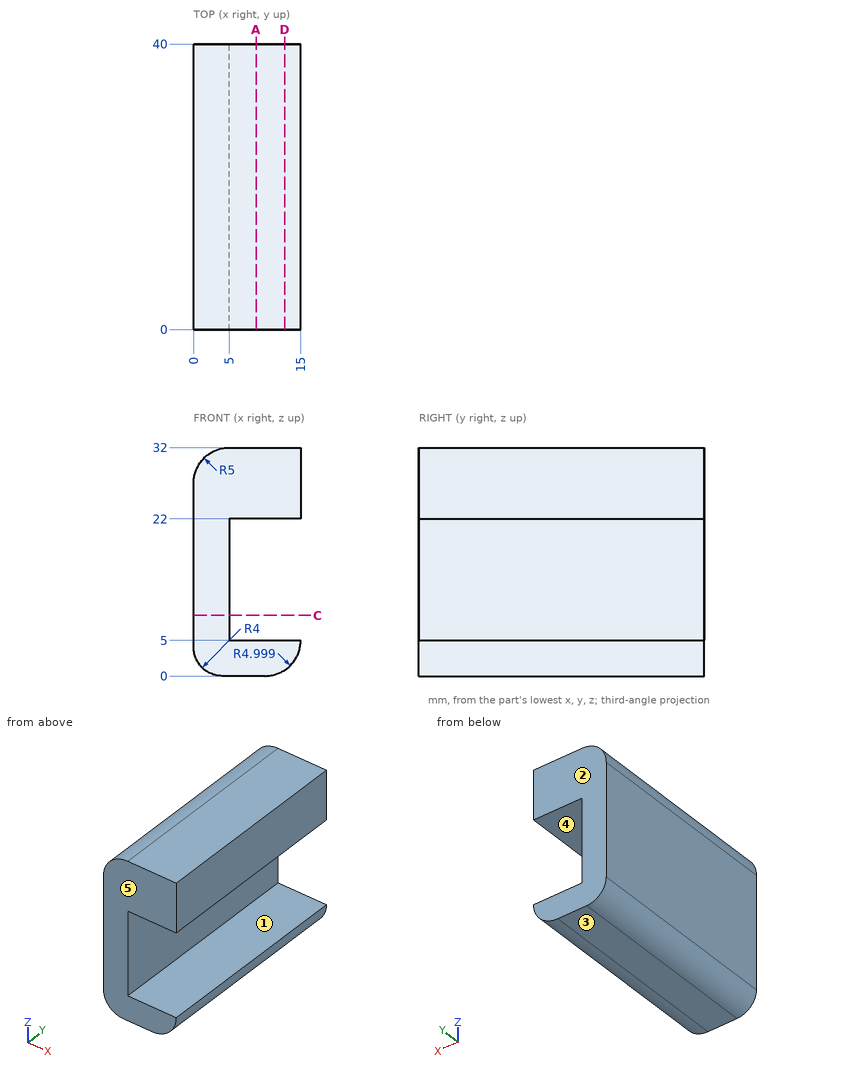
Design review of the part shown in the three views and the two pictorial views. Dimensions are in mm from the part's minimum x, y and z. A direction names the side the tool comes from. Coordinates: 2 decimals unless noted, no trailing zeros. Order: outer loops, then holes, each group sorted by start corner. A loop starts at its lowest first (then second) coordinate and runs counter-clockwise, first axis right, second up. Notation, with made-up numbers: (-29.5, 53) - (10.5, 53) arc R9 ccw to (10.5, 69) - close; hole circle Ø8 at (83, 15.5). An arc over 180 degrees is marked (long way). Answer as CSV lines item,"result". Start each with the question number.
1) To check wall thickness, follow line 1 along Z through (x, y) = (5.25, 7.5); line 2 along Z through (x, y) = (11, 31); line 3 along X through (y, z) = (27, 19). State the ranges of each line that lie inside material, in increasing order. Write a range as [from, to].
2) Insertion check: P1, Ø10, axis at y = 12.5, z = 16.5, coming from the +X side; P2, Ø13.5, axis at y = 23, z = 11, coming from the +X side. Each pin has a flat end and moves straight along its axis. Give the tip position at first contact, or say it passes through.
3) Draft analysis for pull direction Z (two halves, no side actions). For the marked faces 3, 4 and 5, state which applies: +Z half, -Z half, draft (parallel to the pull), parting line (faces both ways), or undercut.
4) Add section A-A (x = 8.75). State the section outline as (y, z) points, then the cut area to 3 significant figures.
5) Add section C-C (z = 8.5). State the section outline as (x, y) points.
6) Machinability: for the marked faces 1 and 2, which of the approach directions +Z, -Z, +X, -X, +Y, -Y give a long, thin tool a straight path to every point of the face, cutting with its end or side? Answer none if there is none.
7) Add section D-D (x = 12.75). State the section outline as (y, z) points, then the cut area to 3 significant figures.
Result:
1,line 1,"[0, 5], [22, 32]"
1,line 2,"[0.1, 5], [22, 32]"
1,line 3,"[0, 5]"
2,P1,"x = 5"
2,P2,"x = 15"
3,face 3,"-Z half"
3,face 4,"undercut"
3,face 5,"draft"
4,outline,"(0, 0) - (40, 0) - (40, 5) - (0, 5) - close; (0, 22) - (40, 22) - (40, 32) - (0, 32) - close"
4,area,"600 mm^2"
5,outline,"(0, 0) - (5, 0) - (5, 40) - (0, 40) - close"
6,face 1,"+X, +Y, -Y"
6,face 2,"+Z, -Z, +X, -X, +Y"
7,outline,"(0, 0.82) - (40, 0.82) - (40, 5) - (0, 5) - close; (0, 22) - (40, 22) - (40, 32) - (0, 32) - close"
7,area,"567 mm^2"
